Work out the finished part from the listing and answer in its coordinate system (mm). Face numbers are marked on the shaded views. A direction names the side the tool comes from. Round coordinates to 2 decimals unless told otherwise and drop trailing zeros. Order: outer loops, then holes, each group sorted by start corner. A loop starts at its lowest first (then second) coordinate and runs counter-clockwise, first axis right, second up. Notation, with made-up numbers: (57.5, 0) - (88.5, 0) arc R26 ccw to (88.5, 39) - close; hole circle Ø10 at (-12.5, 83). An arc over 180 degrees is marked (long way). One line per question, with ' | ' between items. Start each with the question number.
from build123d import *

# Parameters (mm, degrees)
SKIZZE1_W                       = 15
SKIZZE1_H                       = 7.5
AUFSATZ_LINEAR_AUSTRAGEN1_DEPTH = 20
AUFSATZ_LINEAR_AUSTRAGEN2_DEPTH = 15
AUFSATZ_LINEAR_AUSTRAGEN3_DEPTH = 10


with BuildPart() as part:
    # Skizze1 → Aufsatz-Linear austragen1 (new body)
    with BuildSketch(Plane(origin=(0, 0, 0), x_dir=(1, 0, 0), z_dir=(0, 1, 0))):
        Rectangle(SKIZZE1_W, SKIZZE1_H)
        Polygon((-5, 1), (-5, 3.25), (5, 3.25), (5, 1), (7, 1), (7, -1), (5, -1), (5, -3.25), (-5, -3.25), (-5, -1), (-7, -1), (-7, 1), align=None, mode=Mode.SUBTRACT)
    extrude(amount=AUFSATZ_LINEAR_AUSTRAGEN1_DEPTH)

    # Skizze2 → Aufsatz-Linear austragen2 (add)
    with BuildSketch(Plane.ZY.offset(7.5)):
        Polygon((3.75, 0), (3.75, 20), (3.25, 20), (13.25, 37.320508076), (13.683012702, 37.070508076), align=None)
    extrude(amount=-AUFSATZ_LINEAR_AUSTRAGEN2_DEPTH)

    # Skizze4 → Aufsatz-Linear austragen3 (add)
    with BuildSketch(Plane.ZY.offset(7.5)):
        Polygon((10.75, 32.990381057), (11.183012702, 32.740381057), (13.683012702, 37.070508076), (13.25, 37.320508076), align=None)
    aufsatz_linear_austragen3 = extrude(amount=AUFSATZ_LINEAR_AUSTRAGEN3_DEPTH)

    # Spiegeln3: Aufsatz-Linear austragen3 across plane
    add(aufsatz_linear_austragen3.mirror(Plane(origin=(0, 0, 0), x_dir=(0, 0, 1), z_dir=(1, 0, 0))))


solid = part.part
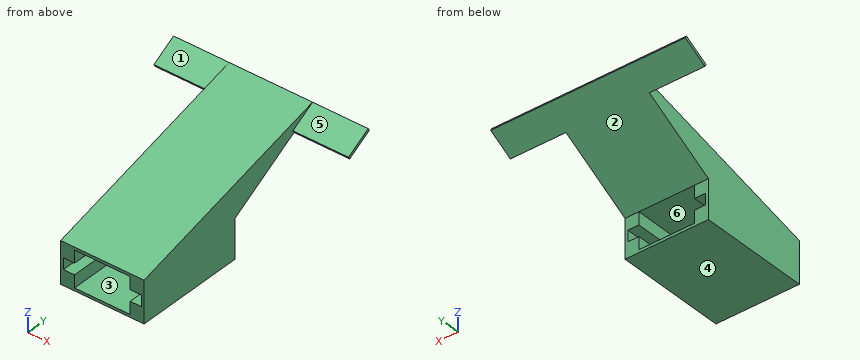
1) Determine the mould class of the marked faces 4, 5 and 6 for opening direction Z: released by +Z, released by -Z, zero draft, split by the parting line, or undercut.
2) Section D-D on z = 0.5 is taken. Give the vertices of the cut face in (x, y), and give its area (3 significant figures).
3) Section C-C on y = 6.5 is taken. Give the vertices of the cut face in (x, z), and give its area (3 significant figures).
4) Section B-B on x = 1 is taken. Give the vertices of the cut face in (y, z).
5) Flat-ended cylindrical pins translate along their axes: pin 1 (0.6 mm diameter, centred on y = 10.5, z = 0.5, fed in from -X); pin 2 (5 mm diameter, centred on x = -1, y = 8, fed in from +Z); pin 3 (1 mm diameter, centred on y = 12.5, z = -0.5, fed in from +X); pin 4 (10 mm diameter, centred on y = 27.5, z = 1.5, fed in from -X). Find the tip coordinate at first contact, or state that the pin passes through.
6) Section A-A on z = -1.5 is taken. Give the vertices of the cut face in (x, y).
7) For the marked faces 1, 2 and 3, determine the directions among +Z, -Z, +X, -X, +Y, -Y from which every point of the face is accessible in a straight line to the end or side of a thin tool.
8) Straight lines are drawn through the part: line 1 (X direction, y = 16, z = -2.5); line 2 (X direction, y = 5.5, z = 0.5); line 3 (Y direction, x = 7, z = -2). For each, find the intervals that lie inside material, in ascending order.
Recorded:
1) face 4: released by -Z | face 5: released by +Z | face 6: undercut
2) outline: (-7.5, 0) - (-7, 0) - (-7, 20) - (-7.5, 20) - close; (7, 0) - (7.5, 0) - (7.5, 20) - (7, 20) - close | area: 20.0 mm²
3) outline: (-7.5, -3.75) - (7.5, -3.75) - (7.5, 5.49) - (-7.5, 5.49) - close; hole (-7, -1) - (-5, -1) - (-5, -3.25) - (5, -3.25) - (5, -1) - (7, -1) - (7, 1) - (5, 1) - (5, 3.25) - (-5, 3.25) - (-5, 1) - (-7, 1) - close | area: 65.6 mm²
4) outline: (0, -3.75) - (20, -3.75) - (20, -3.25) - (0, -3.25) - close; (0, 3.25) - (20, 3.25) - (37.32, 13.25) - (37.07, 13.68) - (0, 3.75) - close
5) pin 1: stops at x = -7.5 | pin 2: stops at z = 6.56 | pin 3: stops at x = 7.5 | pin 4: passes through
6) outline: (-7.5, 0) - (-5, 0) - (-5, 20) - (-7.5, 20) - close; (5, 0) - (7.5, 0) - (7.5, 20) - (5, 20) - close
7) face 1: +Z, -X, -Y | face 2: -Z, +X, -X, +Y | face 3: +Y, -Y
8) line 1: x = -7.5 to -5, 5 to 7.5 | line 2: x = -7.5 to -7, 7 to 7.5 | line 3: y = 0 to 20
